Autodesk Inventor part; units mm, degrees
ref_plane "YZ Plane" through (0, 0, 0) normal (1, 0, 0) x (0, 1, 0)
ref_plane "XZ Plane" through (0, 0, 0) normal (0, 1, 0) x (-1, 0, 0)
ref_plane "XY Plane" through (0, 0, 0) normal (0, 0, 1) x (1, 0, 0)
sketch "Náčrt1" plane through (0, 0, 0) normal (0, 0, 1) x (1, 0, 0)
  line L0 (-10, 10) -> (10, 10)
  line L1 (10, 10) -> (10, -10)
  line L2 (10, -10) -> (-10, -10)
  line L3 (-10, -10) -> (-10, 10)
  point P0 (0, 0)
  dimension "d0" = 20
  dimension "d1" = 20
  dimension "d2" = 10
  dimension "d3" = 10
extrude "Vysunutí1" add sketch "Náčrt1" along normal blind 0.5
sketch "Náčrt2" plane through (0, 0, 0.5) normal (0, 0, 1) x (1, 0, 0)
  circle A0 centre (-5, 5) radius 2
  line L0 (10, 10) -> (-10, 10)
  line L1 (-10, 10) -> (-10, -10)
  point P0 (0, 0)
  dimension "d6" = 4
  dimension "d7" = 5
  dimension "d8" = 5
extrude "Vysunutí2" cut sketch "Náčrt2" against normal blind 0.5
pattern_linear "Obdélníkové pole1" count 2 spacing 10 along (1, 0, 0) count 2 spacing 10 along (0, -1, 0) of "Vysunutí2"
fillet "Zaoblení1" radius 1 1 edges at (10, 10, 0.25)
fillet "Zaoblení2" radius 1 2 edges at (-10, 10, 0.25) (-10, -10, 0.25)
fillet "Zaoblení3" radius 1 1 edges at (10, -10, 0.25)
properties part number "4076"
Design review of the part built by this model. Coordinates are the model's own, in mm. Give positions to 0.01 mm unless a question says otherwise; leave off trailing zeros. Order: outer loops, then holes, each group sorted by start corner. A loop starts at its lowest first (then second) coordinate and runs counter-clockwise, first axis right, second up.
1. Add section C-C, the plane z = 0.4. State the section outline as (x, y) points.
Solution:
outline: (-10, -9) arc R1 ccw to (-9, -10) - (9, -10) arc R1 ccw to (10, -9) - (10, 9) arc R1 ccw to (9, 10) - (-9, 10) arc R1 ccw to (-10, 9) - close; hole circle Ø4 at (-5, -5); hole circle Ø4 at (-5, 5); hole circle Ø4 at (5, -5); hole circle Ø4 at (5, 5)
2. To check wall thickness, follow L1, parallel to Y at x = -5, z = 0.2; L2, parallel to X at y = -6.25, z = 0.15; L3, parallel to Y at x = 5.75, z = 0.1. State the ranges of each line that lie inside material, in increasing order.
Solution:
L1: y = -10 to -7, -3 to 3, 7 to 10
L2: x = -10 to -6.56, -3.44 to 3.44, 6.56 to 10
L3: y = -10 to -6.85, -3.15 to 3.15, 6.85 to 10
3. Mouldability with a two-part tool opening along X and no side actions: class faces 1 (the cylindrical face through (9.699, -9.715, 0.254)), 2 (the cylindrical face through (-9.699, 9.715, 0.254)), 3 (the cylindrical face through (3.4, -6.2, 0.3)), 4 (the cylindrical face through (-6.998, 5.088, 0.254)) as +X half, -X half, draft (parallel to the pull), parting line (faces both ways), or undercut.
Solution:
face 1: +X half
face 2: -X half
face 3: undercut
face 4: undercut
4. Add section A-A, the plane y = -5. State the section outline as (x, z) points, then the cut area to 3 significant figures.
Solution:
outline: (-10, 0) - (-7, 0) - (-7, 0.5) - (-10, 0.5) - close; (-3, 0) - (3, 0) - (3, 0.5) - (-3, 0.5) - close; (7, 0) - (10, 0) - (10, 0.5) - (7, 0.5) - close
area: 6.00 mm2
5. For pin 1 Ø2.5 at (x, y) = (5, -5) entering from +Z; pin 2 Ø5 at (x, y) = (5, 5) entering from +Z, all flat-tipped, find the tip position at first contact; note any pin that passes through.
Solution:
pin 1: passes through
pin 2: stops at z = 0.5
